from build123d import *

# Parameters (mm, degrees)
ESQUISSE1_W             = 20
ESQUISSE1_H             = 16
BOSS_EXTRU_1_DEPTH      = 11.5
TROU_TARAUD_M61_D       = 5
PER_AGE1_D              = 1
PER_AGE1_DEPTH          = 4.5
PER_AGE1_CBORE_D        = 2
PER_AGE1_CBORE_DEPTH    = 2
TROU_TARAUD_M2_51_D     = 2.05
TROU_TARAUD_M2_51_DEPTH = 4.5
TROU_TARAUD_M2_51_TIP   = 0.615882135
D_GAGEMENT_M61_D        = 6.6
ESQUISSE10_W            = 11.487199582
ESQUISSE10_H            = 2
ENL_V_MAT_EXTRU_1_DEPTH = 25.916109247
TROU_TARAUD_M21_D       = 1.6
TROU_TARAUD_M21_DEPTH   = 3
D_GAGEMENT_M21_D        = 2.4
D_GAGEMENT_M21_DEPTH    = 6.5
CHANFREIN1_SIZE         = 0.2


with BuildPart() as part:
    # Esquisse1 → Boss.-Extru.1 (new body)
    with BuildSketch(Plane.XY):
        with Locations((5.25, 0)):
            Rectangle(ESQUISSE1_W, ESQUISSE1_H)
    extrude(amount=BOSS_EXTRU_1_DEPTH)

    # Trou taraudé M61 (through all)
    with Locations(Plane.XY.offset(11.5)):
        with Locations((0, 0)):
            Hole(TROU_TARAUD_M61_D / 2)

    # Perçage1
    with Locations(Plane(origin=(0, -8, 0), x_dir=(-1, 0, 0), z_dir=(0, -1, 0))):
        with Locations((2.25, -9)):
            CounterBoreHole(PER_AGE1_D / 2, PER_AGE1_CBORE_D / 2, PER_AGE1_CBORE_DEPTH, depth=PER_AGE1_DEPTH)

    # Trou taraudé M2.51
    with Locations(Plane(origin=(0, -8, 0), x_dir=(-1, 0, 0), z_dir=(0, -1, 0))):
        with Locations((1.25, -6.5)):
            Hole(TROU_TARAUD_M2_51_D / 2, depth=TROU_TARAUD_M2_51_DEPTH)
            with Locations((0, 0, -(TROU_TARAUD_M2_51_DEPTH + TROU_TARAUD_M2_51_TIP / 2))):  # 118° drill point
                Cone(0, TROU_TARAUD_M2_51_D / 2, TROU_TARAUD_M2_51_TIP, mode=Mode.SUBTRACT)

    # Dégagement M61 (through all)
    with Locations(Plane(origin=(0, -8, 0), x_dir=(-1, 0, 0), z_dir=(0, -1, 0))):
        with Locations((-6.75, -7.5)):
            Hole(D_GAGEMENT_M61_D / 2)

    # Esquisse10 → Enlèv. mat.-Extru.1 (cut, through all)
    with BuildSketch(Plane.XZ.offset(8)):
        with Locations((12.493599791, 7.5)):
            Rectangle(ESQUISSE10_W, ESQUISSE10_H)
    extrude(amount=-ENL_V_MAT_EXTRU_1_DEPTH, mode=Mode.SUBTRACT)

    # Trou taraudé M21
    with Locations(Plane.XY.offset(11.5)):
        with Locations((13.25, 0)):
            Hole(TROU_TARAUD_M21_D / 2, depth=TROU_TARAUD_M21_DEPTH)

    # Dégagement M21
    with Locations(Plane(origin=(0, 0, 0), x_dir=(-1, 0, 0), z_dir=(0, 0, -1))):
        with Locations((-13.25, 0)):
            Hole(D_GAGEMENT_M21_D / 2, depth=D_GAGEMENT_M21_DEPTH)

    # Chanfrein1
    chanfrein1_edges = [part.edges().sort_by_distance(p)[0] for p in [
        (15.25, 0, 11.5),
        (5.25, 8, 11.5),
        (15.25, 8, 3.25),
        (15.25, -8, 3.25),
        (-4.75, 0, 11.5),
        (5.25, 8, 0),
        (15.25, 0, 0),
        (5.25, -8, 0),
        (-4.75, 0, 0),
        (5.25, -8, 11.5),
        (-4.75, 8, 5.75),
        (15.25, 8, 10),
        (15.25, -8, 10),
        (-4.75, -8, 5.75),
    ]]
    chamfer(chanfrein1_edges, length=CHANFREIN1_SIZE)


solid = part.part
Read the model definition and answer for the solid it produces. Units are mm, in the model's axes. A direction names the side the tool comes from. Coordinates: 2 decimals unless noted, no trailing zeros. Loops run counter-clockwise (first coordinate to the right, second up) from the corner with the lowest first, then second, coordinate; pieces in that order, holes last. Notation, with made-up numbers: (-28.75, 16.5) - (-15.75, 16.5) arc R22 ccw to (-15.75, 43.5) - close; hole circle Ø4 at (4.25, 21). An arc over 180 degrees is marked (long way). Answer in a Markdown table with one row per item.
Q1. Straight lines are drawn through the part: line 1 along Y through (x, z) = (0, 8.75); line 2 along X through (y, z) = (1.5, 6.25); line 3 along X through (y, z) = (-4.2, 9). For each, find the intervals that lie inside material, in ascending order. Write a range as [from, to].
Here are the results:
| item | result |
|---|---|
| line 1 | y = [-8, -2.5], [2.5, 8] |
| line 2 | x = [-4.75, -2], [2, 3.7], [9.8, 15.25] |
| line 3 | x = [-4.75, -2.75], [-1.75, 3.81], [9.69, 15.25] |
Q2. Given P1, Ø0.6, axis at x = -2, z = 9, coming from the -Y side; P2, Ø1.9, axis at x = 13.25, y = 0, coming from the +Z side; P3, Ø6, axis at x = 6.75, z = 7.5, coming from the -Y side; P4, Ø1.8, axis at x = 13.25, y = 0, coming from the -Z side, each flat-ended and moving along its own axis, determine where each tip first touches the part or whether it passes through.
Here are the results:
| item | result |
|---|---|
| P1 | stops at y = -6 |
| P2 | stops at z = 11.5 |
| P3 | passes through |
| P4 | stops at z = 8.5 |
Q3. For faces 1 (the cylindrical face through (3.453, 0.112, 7.369)), 2 (the flat face through (11.9, -0.1, 6.5)), 3 (the flat face through (-3, -6, 9)), 4 (the cylindrical face through (14.395, 0.36, 3.296)), determine the directions among +Z, -Z, +X, -X, +Y, -Y from which every point of the face is accessible in a straight line to the end or side of a thin tool.
Here are the results:
| item | result |
|---|---|
| face 1 | +Y, -Y |
| face 2 | +X, +Y, -Y |
| face 3 | -Y |
| face 4 | -Z |
Q4. Find section C-C on y = 0. Write down the section's boundary in (x, z).
Here are the results:
| item | result |
|---|---|
| outline | (-4.75, 0.2) - (-4.55, 0) - (-2.5, 0) - (-2.5, 11.5) - (-4.55, 11.5) - (-4.75, 11.3) - close; (2.5, 0) - (12.05, 0) - (12.05, 6.5) - (9.89, 6.5) arc R3.3 cw (long way) to (9.89, 8.5) - (12.45, 8.5) - (12.45, 11.5) - (2.5, 11.5) - close; (14.05, 8.5) - (15.25, 8.5) - (15.25, 11.3) - (15.05, 11.5) - (14.05, 11.5) - close; (14.45, 0) - (15.05, 0) - (15.25, 0.2) - (15.25, 6.5) - (14.45, 6.5) - close |
Q5. Find section B-B on y = -2. Write down the section's boundary in (x, z).
Here are the results:
| item | result |
|---|---|
| outline | (-4.75, 0.2) - (-4.55, 0) - (-1.5, 0) - (-1.5, 11.5) - (-4.55, 11.5) - (-4.75, 11.3) - close; (1.5, 0) - (15.05, 0) - (15.25, 0.2) - (15.25, 6.5) - (9.89, 6.5) arc R3.3 cw (long way) to (9.89, 8.5) - (15.25, 8.5) - (15.25, 11.3) - (15.05, 11.5) - (1.5, 11.5) - close |
Q6. The mould has two halves that part along Z. Classify faces 5 (the flat face through (12, 0, 8.5)), 6 (the flat face through (5, 8, 4)), 7 (the flat face through (5, 0, 11.5)), 8 (the flat face through (5, 0, 0)): pulls with the +Z half, pulls with the -Z half, needs draft (parallel to the pull), parting line crosses it, or undercut.
Here are the results:
| item | result |
|---|---|
| face 5 | undercut |
| face 6 | needs draft |
| face 7 | pulls with the +Z half |
| face 8 | pulls with the -Z half |
Q7. Find section D-D on x = 13.25. Write down the section's boundary in (y, z).
Here are the results:
| item | result |
|---|---|
| outline | (-8, 0.2) - (-7.8, 0) - (-1.2, 0) - (-1.2, 6.5) - (-8, 6.5) - close; (-8, 8.5) - (-0.8, 8.5) - (-0.8, 11.5) - (-7.8, 11.5) - (-8, 11.3) - close; (0.8, 8.5) - (8, 8.5) - (8, 11.3) - (7.8, 11.5) - (0.8, 11.5) - close; (1.2, 0) - (7.8, 0) - (8, 0.2) - (8, 6.5) - (1.2, 6.5) - close |
Q8. Find section A-A on x = 6.75. Write down the section's boundary in (y, z).
Here are the results:
| item | result |
|---|---|
| outline | (-8, 0.2) - (-7.8, 0) - (7.8, 0) - (8, 0.2) - (8, 4.2) - (-8, 4.2) - close; (-8, 10.8) - (8, 10.8) - (8, 11.3) - (7.8, 11.5) - (-7.8, 11.5) - (-8, 11.3) - close |
